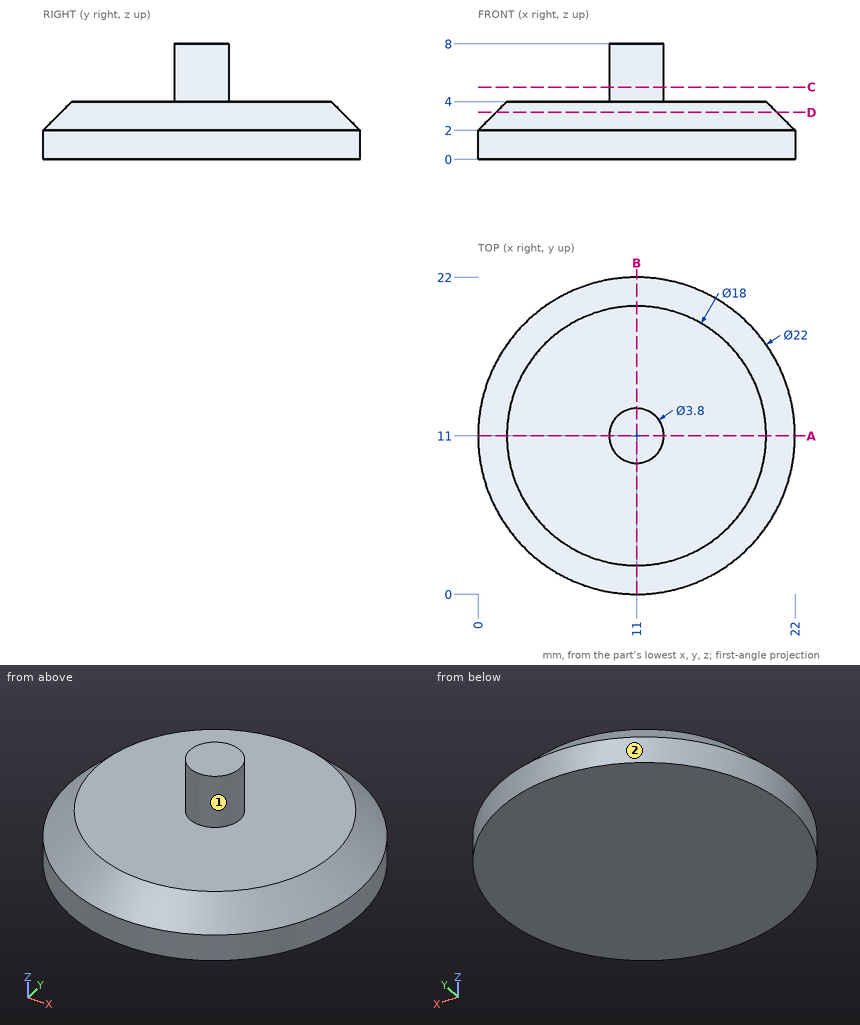
Design review of the part shown in the three views and the two pictorial views. Dimensions are in mm from the part's minimum x, y and z. A direction names the side the tool comes from. Coordinates: 2 decimals unless noted, no trailing zeros. Order: outer loops, then holes, each group sorted by start corner. A loop starts at its lowest first (then second) coordinate and runs counter-clockwise, first axis right, second up.
Item 1: Take a section at D-D, the plane z = 3.25. Write out the cut boundary in (x, y).
Item 2: For the marked faces 1 and 2, list the 3-axis set-ups (+Z, -Z, +X, -X, +Y, -Y) from which the entire face can be reached by the end or side of a thin tool; tool diameter is ignored.
Item 3: Take a section at C-C, the plane z = 5. Write out the cut boundary in (x, y), then the cut area to 3 significant figures.
Item 4: Take a section at A-A, the plane y = 11. Write out the cut boundary in (x, z), then the cut area to 3 significant figures.
Item 5: For pin 1 Ø2 at (y, z) = (17.5, 2.5) entering from -X; pin 2 Ø4 at (x, y) = (5, 5) entering from +Z; pin 3 Ø1 at (x, z) = (9.5, 5) entering from +Y, all flat-tipped, find the tip position at first contact; note any pin that passes through.
Item 6: For line 1 (Z direction, x = 14, y = 14); line 2 (X direction, y = 10.75, z = 1.5); line 3 (X direction, y = 11.75, z = 2.5), list the stretches that pass through material, from the lowest coordinate up.
The answers:
1. outline: circle Ø19.5 at (11, 11)
2. face 1: +Z
2. face 2: +Z, -Z
3. outline: circle Ø3.8 at (11, 11)
3. area: 11.3 mm2
4. outline: (0, 0) - (22, 0) - (22, 2) - (20, 4) - (12.9, 4) - (12.9, 8) - (9.1, 8) - (9.1, 4) - (2, 4) - (0, 2) - close
4. area: 99.2 mm2
5. pin 1: stops at x = 1.55
5. pin 2: stops at z = 4
5. pin 3: stops at y = 12.62
6. line 1: z = 0 to 4
6. line 2: x = 0 to 22
6. line 3: x = 0.53 to 21.47
